Build history of the part. All positions in model axes, mm. A direction names the side the tool comes from. Give positions to 0.01 mm unless a question says otherwise; leave off trailing zeros. Write each loop counter-clockwise with the first axis right and the second up, starting at its lowest first coordinate (ties: lowest second). Pieces come first, ordered by that corner, then holes.
from build123d import *

# Parameters (mm, degrees)
ESBO_O1_W                     = 30
ESBO_O1_H                     = 12
RESSALTO_EXTRUS_O1_DEPTH      = 7.5
RESSALTO_EXTRUS_O1_DEPTH_BACK = 7.5
ESBO_O1_3_W                   = 57.5
ESBO_O1_3_H                   = 12
RESSALTO_EXTRUS_O2_DEPTH      = 4
RESSALTO_EXTRUS_O2_DEPTH_BACK = 4
RESSALTO_EXTRUS_O3_DEPTH      = 3
RESSALTO_EXTRUS_O4_DEPTH      = 3
ESBO_O1_9_W                   = 30
ESBO_O1_9_H                   = 12
RESSALTO_EXTRUS_O6_DEPTH      = 7.5
RESSALTO_EXTRUS_O6_DEPTH_BACK = 7.5
ESBO_O5_R                     = 2.75
CORTE_EXTRUS_O1_DEPTH         = 72
ESBO_O5_8_R                   = 4.5
ESBO_O5_8_R_2                 = 2.75
RESSALTO_EXTRUS_O7_DEPTH      = 2.5


with BuildPart() as part:
    # Esbo_o1 → Ressalto-extrus_o1 (new body, two sides)
    with BuildSketch(Plane.XY) as ressalto_extrus_o1_sk:
        with Locations((-40.5, -0.65)):
            Rectangle(ESBO_O1_W, ESBO_O1_H)
    extrude(amount=RESSALTO_EXTRUS_O1_DEPTH)
    extrude(ressalto_extrus_o1_sk.sketch, amount=-RESSALTO_EXTRUS_O1_DEPTH_BACK)

    # Esbo_o1_3 → Ressalto-extrus_o2 (add, two sides)
    with BuildSketch(Plane.XY) as ressalto_extrus_o2_sk:
        with Locations((3.25, -0.65)):
            Rectangle(ESBO_O1_3_W, ESBO_O1_3_H)
    extrude(amount=RESSALTO_EXTRUS_O2_DEPTH)
    extrude(ressalto_extrus_o2_sk.sketch, amount=-RESSALTO_EXTRUS_O2_DEPTH_BACK)

    # Esbo_o2 → Ressalto-extrus_o3 (add)
    with BuildSketch(Plane(origin=(-55.5, -6.65, -7.5), x_dir=(-1, 0, 0), z_dir=(0, -1, 0))):
        Polygon((-37.6, -6.5), (-37.6, -7.5), (-37.6, -8.5), (-33.6, -8.5), (-33.6, -6.5), align=None)
        Polygon((-7.6, -7.5), (-7.6, -8.5), (-3.6, -8.5), (-3.6, -7.5), (-3.6, -6.5), (-7.6, -6.5), align=None)
    extrude(amount=RESSALTO_EXTRUS_O3_DEPTH)

    # Esbo_o3 → Ressalto-extrus_o4 (add)
    with BuildSketch(Plane(origin=(-55.5, 5.35, -7.5), x_dir=(-1, 0, 0), z_dir=(0, -1, 0))):
        Polygon((-37.6, -6.5), (-37.6, -7.5), (-37.6, -8.5), (-33.6, -8.5), (-33.6, -6.5), align=None)
        Polygon((-7.6, -7.5), (-7.6, -8.5), (-3.6, -8.5), (-3.6, -7.5), (-3.6, -6.5), (-7.6, -6.5), align=None)
    extrude(amount=-RESSALTO_EXTRUS_O4_DEPTH)

    # Esbo_o1_9 → Ressalto-extrus_o6 (add, two sides)
    with BuildSketch(Plane.XY) as ressalto_extrus_o6_sk:
        with Locations((-40.5, -0.65)):
            Rectangle(ESBO_O1_9_W, ESBO_O1_9_H)
    extrude(amount=RESSALTO_EXTRUS_O6_DEPTH)
    extrude(ressalto_extrus_o6_sk.sketch, amount=-RESSALTO_EXTRUS_O6_DEPTH_BACK)

    # Esbo_o5 → Corte-extrus_o1 (cut)
    with BuildSketch(Plane(origin=(-55.5, 5.35, -7.5), x_dir=(0, 0, 1), z_dir=(-1, 0, 0))):
        with Locations((7.5, -6.65)):
            Circle(ESBO_O5_R)
    extrude(amount=-CORTE_EXTRUS_O1_DEPTH, mode=Mode.SUBTRACT)

    # Esbo_o5_8 → Ressalto-extrus_o7 (add)
    with BuildSketch(Plane(origin=(-55.5, 5.35, -7.5), x_dir=(0, 0, 1), z_dir=(-1, 0, 0))):
        with Locations((7.5, -6.65)):
            Circle(ESBO_O5_8_R)
        with Locations((7.5, -6.65)):
            Circle(ESBO_O5_8_R_2, mode=Mode.SUBTRACT)
    extrude(amount=RESSALTO_EXTRUS_O7_DEPTH)


solid = part.part
(1) Saw through at C-C, the plane y = -1.3. List the corners of the cut face in (x, z), plus the area to 3 significant figures.
(2) 3-axis set-ups, long thin cutter, end or side, ignore diameter. For faces 1 (the face through (-50, 7, 1)), 2 (the face through (-20, 7, -1)), 3 (the face through (3, -1, -4)): which of +Z, -Z, +X, -X, +Y, -Y reach the whole face in a straight line?
(3) Mould opens along Z. For faces 4 (the face through (-17.9, 7, 0)), 5 (the face through (16.5, -1, 0)), 6 (the face through (3, -1, 4)), 7 (the face through (-20.228, -3.985, -0.596)) say: +Z half, -Z half, draft (parallel to the pull), parting line (faces both ways), or undercut.
(4) Saw through at D-D, the plane z = 5.5. List the corners of the cut face in (x, y).
(5) Saw through at B-B, the plane z = 0. List the corners of the cut face in (x, y), plus the area to 3 significant figures.
(6) Saw through at A-A, the plane x = 1. List the corners of the cut face in (y, z), plus the area to 3 significant figures.
(7) Probe line 1 (Y direction, x = -24.5, z = 0); line 2 (X direction, y = -9, z = -0.5); line 3 (X direction, y = -2.75, z = -6.5). List the from-to ranges inside material, lowest first.
(8) Drop flat-ended pins along their axis: pin 1 (1.5 mm diameter, centred on x = -20, y = 6.5, fed in from +Z); pin 2 (3.5 mm diameter, centred on x = -8, y = 2, fed in from -Z); pin 3 (3 mm diameter, centred on y = 2, z = -3.5, fed in from -X); pin 4 (6 mm diameter, centred on y = -7.5, z = -5, fed in from -X). Give the stop position or say it passes through.
Computed values:
1. outline: (-58, -4.5) - (-55.5, -4.5) - (-55.5, -7.5) - (-25.5, -7.5) - (-25.5, -4) - (32, -4) - (32, 4) - (-25.5, 4) - (-25.5, 7.5) - (-55.5, 7.5) - (-55.5, 4.5) - (-58, 4.5) - (-58, 2.75) - (16.5, 2.75) - (16.5, -2.75) - (-58, -2.75) - close
1. area: 523 mm2
2. face 1: +Z, +X, -X, +Y
2. face 2: -Z, +X, -X, +Y
2. face 3: -Z, +X, +Y, -Y
3. face 4: draft
3. face 5: undercut
3. face 6: +Z half
3. face 7: undercut
4. outline: (-55.5, -6.65) - (-25.5, -6.65) - (-25.5, 5.35) - (-55.5, 5.35) - close
5. outline: (-58, -5.8) - (-55.5, -5.8) - (-55.5, -6.65) - (-51.9, -6.65) - (-51.9, -9.65) - (-47.9, -9.65) - (-47.9, -6.65) - (-21.9, -6.65) - (-21.9, -9.65) - (-17.9, -9.65) - (-17.9, -6.65) - (32, -6.65) - (32, 5.35) - (-17.9, 5.35) - (-17.9, 8.35) - (-21.9, 8.35) - (-21.9, 5.35) - (-47.9, 5.35) - (-47.9, 8.35) - (-51.9, 8.35) - (-51.9, 5.35) - (-55.5, 5.35) - (-55.5, 3.2) - (-58, 3.2) - (-58, 1.45) - (16.5, 1.45) - (16.5, -4.05) - (-58, -4.05) - close
5. area: 711 mm2
6. outline: (-6.65, -4) - (5.35, -4) - (5.35, 4) - (-6.65, 4) - close; hole circle Ø5.5 at (-1.3, 0)
6. area: 72.2 mm2
7. line 1: y = -6.65 to -4.05, 1.45 to 5.35
7. line 2: x = -51.9 to -47.9, -21.9 to -17.9
7. line 3: x = -55.5 to -25.5
8. pin 1: stops at z = 1
8. pin 2: stops at z = -4
8. pin 3: stops at x = -58
8. pin 4: stops at x = -55.5
